from build123d import *

# Parameters (mm, degrees)
F0_R     = 35
F1_DEPTH = 150
F2_R     = 25
F3_DEPTH = 90
F4_R     = 5
F5_DEPTH = 150.001


with BuildPart() as f1:
    # F0 (on Top) → F1 (new body)
    with BuildSketch(Plane.XY):
        Circle(F0_R)
    extrude(amount=F1_DEPTH)

    # F2 (on face) → F3 (cut)
    with BuildSketch(Plane(origin=(0, 0, 0), x_dir=(1, 0, 0), z_dir=(0, 0, -1))):
        Circle(F2_R)
    extrude(amount=-F3_DEPTH, mode=Mode.SUBTRACT)

    # F4 (on face) → F5 (cut, through all)
    with BuildSketch(Plane.XY.offset(150)):
        Circle(F4_R)
    extrude(amount=-F5_DEPTH, mode=Mode.SUBTRACT)


solid = f1.part
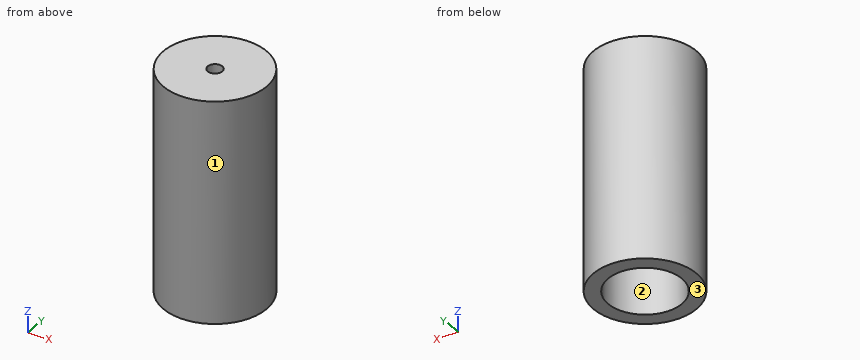
The listing builds one solid part. Answer for the finished solid, in the listing's coordinates (mm). Face numbers are marked on the shaded views. Round coordinates to 2 decimals unless told otherwise and drop trailing zeros. Order: outer loops, then holes, each group sorted by start corner. A loop starts at its lowest first (then second) coordinate and runs counter-clockwise, first axis right, second up. Notation, with made-up numbers: (5.25, 74.25) - (60.25, 74.25) arc R25 ccw to (60.25, 101.25) - close; hole circle Ø9 at (7.5, 48). An arc over 180 degrees is marked (long way). Write item = value, one per line. Start each with the question number.
1) Given pin 1 (1.5 mm diameter, centred on y = -23.5, z = 115.5, fed in from +X); pin 2 (1 mm diameter, centred on y = -26.5, z = 26.5, fed in from +X); pin 3 (3 mm diameter, centred on x = -16.5, z = 73.5, fed in from -Y), each flat-ended and moving along its own axis, determine where each tip first touches the part or whether it passes through.
2) For a pull along X with two mould halves and no side action, classify the marked faces 1, 2 and 3 as released by +X, released by -X, zero draft, split by the parting line, or undercut.
3) Straight lines are drawn through the part: L1, parallel to Y at x = 0, z = 106.5; L2, parallel to Z at x = 18.5, y = 16.5; L3, parallel to X at y = -1, z = 119. For each, find the intervals that lie inside material, in ascending order.
4) Section C-C, the plane z = 65 is taken. Write down the section's boundary in (x, y).
5) Section D-D, the plane x = -28 is taken. Write down the section's boundary in (y, z), plus the area to 3 significant figures.
6) Section A-A, the plane y = 0 is taken. Write down the section's boundary in (x, z), plus the area to 3 significant figures.
Results list:
q1.pin_1 = 26.6
q1.pin_2 = 23.43
q1.pin_3 = -31.62
q2.face_1 = split by the parting line
q2.face_2 = undercut
q2.face_3 = zero draft
q3.L1 = -35 to -5, 5 to 35
q3.L2 = 90 to 150
q3.L3 = -34.99 to -4.9, 4.9 to 34.99
q4.outline = circle Ø70 at (0, 0); hole circle Ø50 at (0, 0)
q5.outline = (-21, 0) - (21, 0) - (21, 150) - (-21, 150) - close
q5.area = 6,300 mm^2
q6.outline = (-35, 0) - (-25, 0) - (-25, 90) - (-5, 90) - (-5, 150) - (-35, 150) - close; (5, 90) - (25, 90) - (25, 0) - (35, 0) - (35, 150) - (5, 150) - close
q6.area = 5,400 mm^2
